Could you check a few things on this model? Use its own coordinates, in mm. A direction names the side the tool comes from. Coordinates: 2 decimals unless noted, no trailing zeros. Loops run counter-clockwise (first coordinate to the right, second up) from the corner with the lowest first, then second, coordinate; pieces in that order, holes last.
from build123d import *

# Parameters (mm, degrees)
MATRIZC1_COUNT = 3


with BuildPart() as part:
    # Croquis1 → Revolución1 (revolve)
    with BuildSketch(Plane.XY, mode=Mode.PRIVATE) as revoluci_n1_sk:
        Polygon((6.371214478, 0), (6.371214478, 18), (7.371214478, 18), (7.371214478, 26), (5.371214478, 26), (5.371214478, 33), (3.371214478, 33), (3.371214478, 0), align=None)
    revolve(revoluci_n1_sk.sketch.rotate(Axis((-9.128785522, 76.373603091, 0), (0, -1, 0)), 180), axis=Axis((-9.128785522, 76.373603091, 0), (0, -1, 0)))

    # Croquis2 → Perforador para roscar para macho de roscar para M2.5x0.451 (revolve, cut)
    with BuildSketch(Plane(origin=(7.216426647, 21.537901264, -2.254781399), x_dir=(-0.13665341811634468, 0, -0.9906189193212089), z_dir=(0, 1, 0))):
        Polygon((0, 0), (0, 10.615882135), (1.025, 10), (1.025, 0), align=None)
    perforador_para_roscar_para_macho_de_ros = revolve(axis=Axis((13.506856785, 21.537901264, -3.122530604), (-0.9906189193212088, 0, 0.13665341811634468)), mode=Mode.SUBTRACT)

    # MatrizC1: Perforador para roscar para macho de roscar para M2.5x0.451 ×3 about axis, 1 skipped
    matrizc1_axis = Axis((-9.128785522, 26, 0), (0, 1, 0))
    add([perforador_para_roscar_para_macho_de_ros.rotate(matrizc1_axis, i * 360 / MATRIZC1_COUNT) for i in range(1, MATRIZC1_COUNT) if i not in (2,)], mode=Mode.SUBTRACT)


solid = part.part
(1) I need wall thicknesses on probe 1 along X at (y, z) = (24, 8.5); probe 2 along Z at (x, y) = (-5.5, 23); probe 3 along X at (y, z) = (13, 6.5). Which ranges of each line are inside material? Lowest first, please.
Answers:
probe 1: x = -23.27 to -18.29, 0.04 to 5.01
probe 2: z = -16.1 to -11.96, 11.96 to 16.1
probe 3: x = -23.2 to -19.81, 1.55 to 4.94
(2) We'd pull the mould along Z, two halves only. Please class faces 1 (the face through (-24, 18, 5)), 2 (the face through (-17.93, 20.52, -11.54)), 3 (the face through (2.38, 29.55, 8.82)): +Z half, -Z half, draft (parallel to the pull), parting line (faces both ways), or undercut.
Answers:
face 1: draft
face 2: undercut
face 3: parting line
(3) Which directions (+Z, -Z, +X, -X, +Y, -Y) give clear straight access to the entire face, cutting with the end or side of a thin tool? Please do faces 4 (the face through (-23.9, 9.1, -4.7)), 5 (the face through (-9, 26, 15)), 6 (the face through (-20, 0, -7)).
Answers:
face 4: -Y
face 5: +Y
face 6: +Z, -Z, +X, -X, -Y
(4) Imagine slicing it at B-B, the plane x = 0.5. Write out the boundary of the cut face in (y, z).
Answers:
outline: (0, -12.15) - (18, -12.15) - (18, -13.4) - (26, -13.4) - (26, -10.84) - (33, -10.84) - (33, -7.97) - (0, -7.97) - close; (0, 7.97) - (33, 7.97) - (33, 10.84) - (26, 10.84) - (26, 13.4) - (18, 13.4) - (18, 12.15) - (0, 12.15) - close
(5) Imagine slicing it at A-A, the plane z = 0. Write out the boundary of the cut face in (x, y), and give its area (3 significant figures).
Answers:
outline: (-25.63, 18) - (-24.63, 18) - (-24.63, 0) - (-21.63, 0) - (-21.63, 33) - (-23.63, 33) - (-23.63, 26) - (-25.63, 26) - close; (3.37, 0) - (6.37, 0) - (6.37, 18) - (7.37, 18) - (7.37, 26) - (5.37, 26) - (5.37, 33) - (3.37, 33) - close
area: 200 mm2
(6) For pin 1 (2 mm diameter, centred on x = -6.5, y = 14, fed in from +Z); pin 2 (10 mm diameter, centred on x = -2.5, y = 25.5, fed in from -Z); pin 3 (8 mm diameter, centred on x = -20.5, y = 28.5, fed in from +Z), each with a flat end and sliding along its axis, tell me the tip position at first contact or that it passes through.
Answers:
pin 1: stops at z = 15.41
pin 2: stops at z = -16.42
pin 3: stops at z = 14.29
(7) Imagine slicing it at C-C, the plane y = 2.5. Write out the boundary of the cut face in (x, z), and give its area (3 significant figures).
Answers:
outline: circle Ø31 at (-9.13, 0); hole circle Ø25 at (-9.13, 0)
area: 264 mm2
(8) Imagine slicing it at D-D, the plane y = 22. Write out the boundary of the cut face in (x, z).
Answers:
outline: (-19.96, -12.45) - (-17.5, -9.28) arc R12.5 cw (long way) to (3.35, -0.8) - (7.32, -1.34) arc R16.5 ccw (long way) to start; (-18.52, -13.57) arc R16.5 ccw to (7.07, -3.16) - (3.1, -2.61) arc R12.5 cw to (-16.06, -10.4) - close
